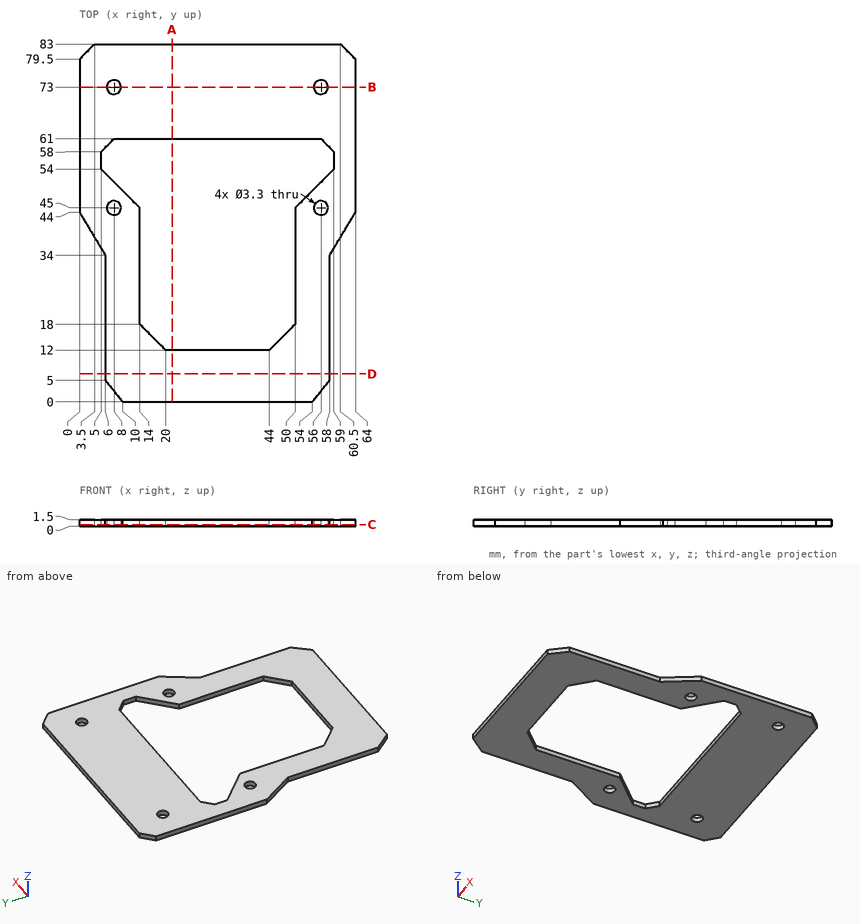
Study the drawing (mm; zero at the part's minimum x, y, z) and answer. Coordinates: 2 decimals unless noted, no trailing zeros. Order: outer loops, then holes, each group sorted by start corner. A loop starts at its lowest first (then second) coordinate and runs counter-clockwise, first axis right, second up. Notation, with made-up numbers: (49, -22.75) -> (98, -22.75) arc R8 cw to (98, -13.75) -> close; hole circle Ø4 at (82, -5.75). An arc over 180 degrees is marked (long way). Answer in a Markdown table with one row per item. Add a question column.
Item 1: Find section D-D (y = 6.5). Write down the section's boundary in (x, z).
Item 2: Each of these flat-tipped pins is pushed along its axis until it touches: P1, Ø2.5, axis at x = 8, y = 45, coming from the +Z side; P2, Ø0.8, axis at y = 32, z = 0.5, coming from the +X side. Where does it stop, or does it pass through?
Item 3: Find section A-A (x = 21.5). Write down the section's boundary in (y, z).
Item 4: Find section C-C (z = 0.4). Write down the section's boundary in (x, y), then the cut area to 3 significant figures.
Item 5: Find section B-B (y = 73). Write down the section's boundary in (x, z).
Item 6: Find the intervals of material crossed by L1, parallel to X at y = 73, z = 0.5; L2, parallel to Y at x = 26, z = 0.3; L3, parallel to X at y = 74.5, z = 0.3, in increasing order. Write a range as from..to.
Result set:
| question | item | result |
|---|---|---|
| 1 | outline | (6, 0) -> (58, 0) -> (58, 1.5) -> (6, 1.5) -> close |
| 2 | P1 | passes through |
| 2 | P2 | stops at x = 58 |
| 3 | outline | (0, 0) -> (12, 0) -> (12, 1.5) -> (0, 1.5) -> close; (61, 0) -> (83, 0) -> (83, 1.5) -> (61, 1.5) -> close |
| 4 | outline | (0, 44) -> (6, 34) -> (6, 5) -> (10, 0) -> (54, 0) -> (58, 5) -> (58, 34) -> (64, 44) -> (64, 79.5) -> (60.5, 83) -> (3.5, 83) -> (0, 79.5) -> close; hole (5, 54) -> (14, 45) -> (14, 18) -> (20, 12) -> (44, 12) -> (50, 18) -> (50, 45) -> (59, 54) -> (59, 58) -> (56, 61) -> (8, 61) -> (5, 58) -> close; hole circle Ø3.3 at (8, 45); hole circle Ø3.3 at (8, 73); hole circle Ø3.3 at (56, 45); hole circle Ø3.3 at (56, 73) |
| 4 | area | 2,850 mm² |
| 5 | outline | (0, 0) -> (6.35, 0) -> (6.35, 1.5) -> (0, 1.5) -> close; (9.65, 0) -> (54.35, 0) -> (54.35, 1.5) -> (9.65, 1.5) -> close; (57.65, 0) -> (64, 0) -> (64, 1.5) -> (57.65, 1.5) -> close |
| 6 | L1 | x = 0..6.35, 9.65..54.35, 57.65..64 |
| 6 | L2 | y = 0..12, 61..83 |
| 6 | L3 | x = 0..7.31, 8.69..55.31, 56.69..64 |
